Verification items for this drawing (mm, ordinates from the low corner). A direction names the side the tool comes from. Coordinates: 2 decimals unless noted, no trailing zeros. Loops run counter-clockwise (first coordinate to the right, second up) from the corner with the lowest first, then second, coordinate; pieces in that order, holes last.
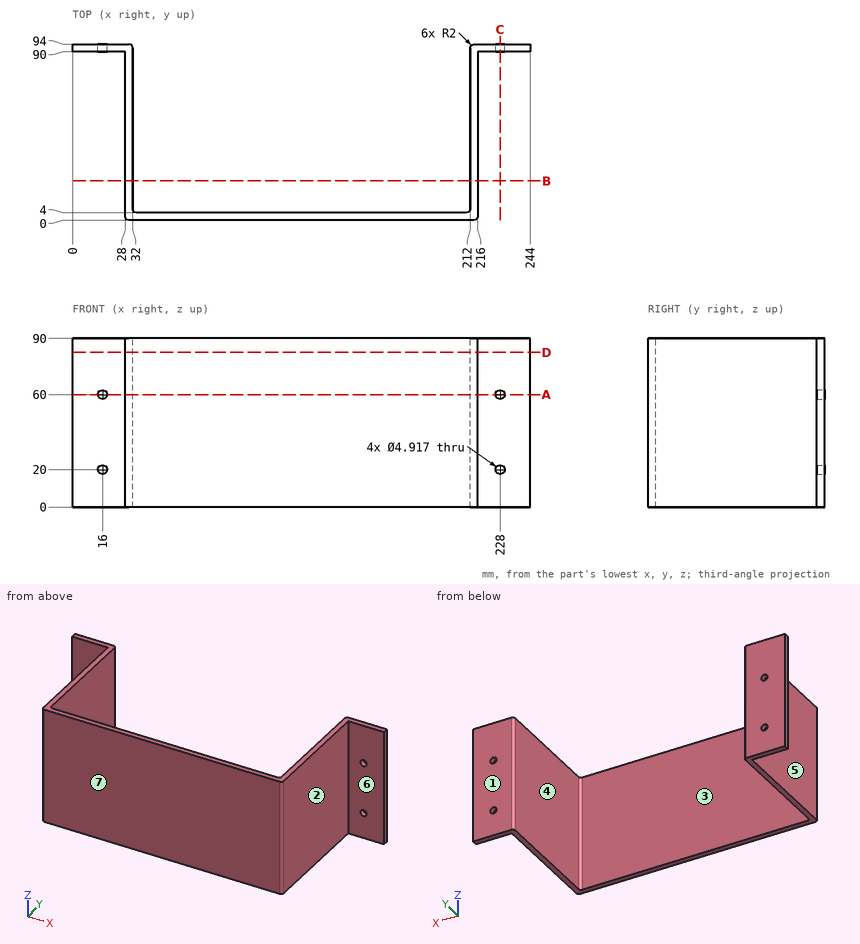
(1) Section check A-A, the plane z = 60. Enter the section's corners in (x, y), plus the area to 3 significant figures.
(2) Section check C-C, the plane x = 228. Enter the section's corners in (y, z), plus the area to 3 significant figures.
(3) Set-up check for the marked faces 4, 5, 6 and 7: record each of +Z, -Z, +X, -X, +Y, -Y from which the full face is reachable in a straight line by a thin tool's end or side.
(4) Section check B-B, the plane y = 21. Enter the section's corners in (x, z), plus the area to 3 significant figures.
(5) Scan lines: line 1 along X through (y, z) = (92, 20); line 2 along Z through (x, y) = (16, 92.85); line 3 along X through (y, z) = (82, 25.5). Record each from-to range of solid material in increasing order.
(6) Draft check along X on the marked faces 1, 2 and 3. Enter one of: pulls with the +X half, pulls with the -X half, needs draft (parallel to the pull), parting line crosses it, or undercut.
(7) Gauge pin test, flat ends, axial feed: P1, Ø14, axis at x = 232.5, z = 40, coming from the -Y side; P2, Ø3, axis at x = 140.5, z = 10, coming from the +Y side; P3, Ø1.5, axis at y = 79, z = 41.5, coming from the +X side. Record the tip position at first contact, or that the pin passes through.
(8) Section check D-D, the plane z = 82.5. Enter the section's corners in (x, y).
Determined:
1. outline: (0, 90) - (13.54, 90) - (13.54, 94) - (0, 94) - close; (18.46, 90) - (28, 90) - (28, 2) arc R2 ccw to (30, 0) - (214, 0) arc R2 ccw to (216, 2) - (216, 90) - (225.54, 90) - (225.54, 94) - (214, 94) arc R2 ccw to (212, 92) - (212, 6) arc R2 cw to (210, 4) - (34, 4) arc R2 cw to (32, 6) - (32, 92) arc R2 ccw to (30, 94) - (18.46, 94) - close; (230.46, 90) - (244, 90) - (244, 94) - (230.46, 94) - close
1. area: 1,650 mm2
2. outline: (90, 0) - (94, 0) - (94, 17.54) - (90, 17.54) - close; (90, 22.46) - (94, 22.46) - (94, 57.54) - (90, 57.54) - close; (90, 62.46) - (94, 62.46) - (94, 90) - (90, 90) - close
2. area: 321 mm2
3. face 4: +Z, -Z, +Y
3. face 5: +Z, -Z, -X, -Y
3. face 6: +Z, -Z, +X, -Y
3. face 7: +Z, -Z, +X, -X, -Y
4. outline: (28, 0) - (32, 0) - (32, 90) - (28, 90) - close; (212, 0) - (216, 0) - (216, 90) - (212, 90) - close
4. area: 720 mm2
5. line 1: x = 0 to 13.54, 18.46 to 32, 212 to 225.54, 230.46 to 244
5. line 2: z = 0 to 17.54, 22.46 to 57.54, 62.46 to 90
5. line 3: x = 28 to 32, 212 to 216
6. face 1: needs draft
6. face 2: pulls with the +X half
6. face 3: undercut
7. P1: stops at y = 90
7. P2: stops at y = 4
7. P3: stops at x = 216
8. outline: (0, 90) - (28, 90) - (28, 2) arc R2 ccw to (30, 0) - (214, 0) arc R2 ccw to (216, 2) - (216, 90) - (244, 90) - (244, 94) - (214, 94) arc R2 ccw to (212, 92) - (212, 6) arc R2 cw to (210, 4) - (34, 4) arc R2 cw to (32, 6) - (32, 92) arc R2 ccw to (30, 94) - (0, 94) - close
